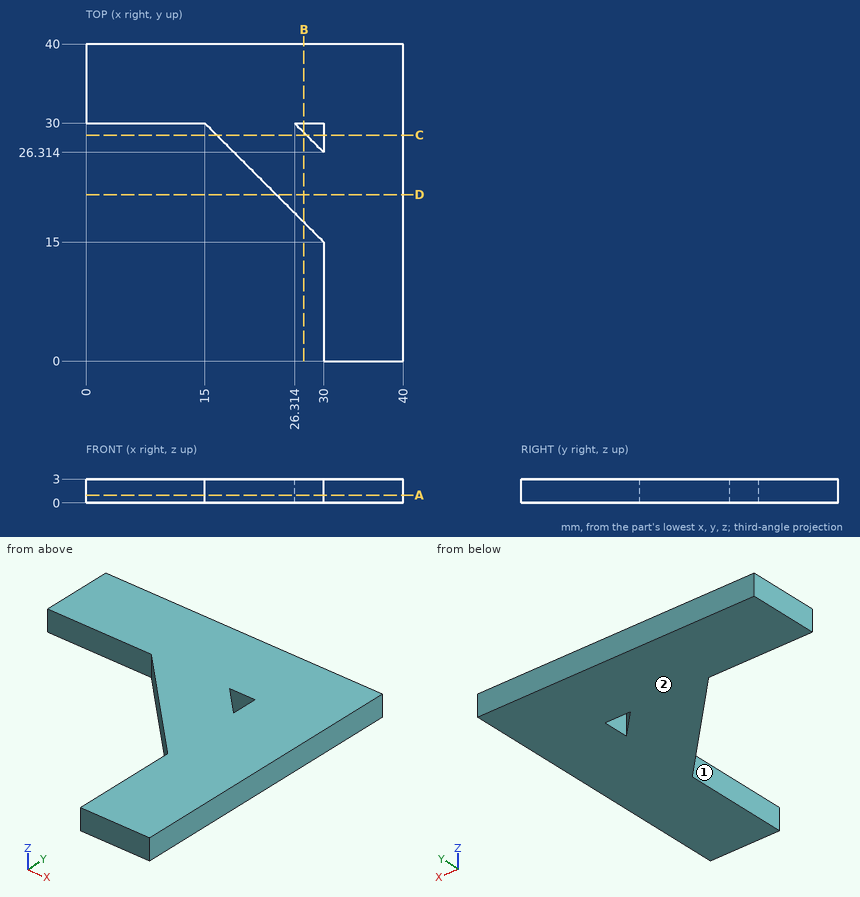
Could you check a few things on this drawing? It's one solid part, dimensions in mm from its lowest x, y, z. A direction names the side the tool comes from. Give positions to 0.01 mm unless a question says otherwise; leave off trailing zeros. Write each loop counter-clockwise with the first axis right and the second up, starting at its lowest first coordinate (ties: lowest second). Pieces come first, ordered by that corner, then holes.
(1) Will these pins go through, and if not, where does the flat tip stop? pin 1 (0.9 mm diameter, centred on x = 8.5, z = 2, fed in from -Y); pin 2 (1.5 mm diameter, centred on x = 35.5, y = 7, fed in from -Z).
Output values:
pin 1: stops at y = 30
pin 2: stops at z = 0
(2) Imagine slicing it at A-A, the plane z = 0.95. Write out the boundary of the cut face in (x, y).
Output values:
outline: (0, 30) - (15, 30) - (30, 15) - (30, 0) - (40, 0) - (40, 40) - (0, 40) - close; hole (26.31, 30) - (30, 26.31) - (30, 30) - close
(3) Imagine slicing it at C-C, the plane y = 28.5. Write out the boundary of the cut face in (x, z).
Output values:
outline: (16.5, 0) - (27.81, 0) - (27.81, 3) - (16.5, 3) - close; (30, 0) - (40, 0) - (40, 3) - (30, 3) - close
(4) Imagine slicing it at D-D, the plane y = 21. Write out the boundary of the cut face in (x, z).
Output values:
outline: (24, 0) - (40, 0) - (40, 3) - (24, 3) - close
(5) On a 3-axis mill with a long thin cutter (end or side, diameter ignored), from which of +Z, -Z, +X, -X, +Y, -Y can I reach the whole of each face in a straight line? I mean the marked faces 1 and 2. Say none if no direction works.
Output values:
face 1: +Z, -Z, -X, -Y
face 2: -Z, +X, -X, +Y, -Y
(6) If I drill on L1, parallel to Y at x = 7, z = 1.7; L2, parallel to X at y = 27, z = 0.4 (1 decimal), over which ranges is the centre line in solid material (lowest first)?
Output values:
L1: y = 30 to 40
L2: x = 18 to 29.3, 30 to 40
(7) Imagine slicing it at B-B, the plane x = 27.5. Write out the boundary of the cut face in (y, z).
Output values:
outline: (17.5, 0) - (28.81, 0) - (28.81, 3) - (17.5, 3) - close; (30, 0) - (40, 0) - (40, 3) - (30, 3) - close
